Could you check a few things on this model? Use its own coordinates, in mm. Round coordinates to 2 decimals unless told otherwise and drop trailing zeros. Loops run counter-clockwise (first coordinate to the right, second up) from the corner with the lowest first, then second, coordinate; pieces in that order, holes last. Notation, with made-up numbers: (31.25, -25) - (69.25, -25) arc R28 ccw to (69.25, 13) - close; hole circle Ø7 at (-30.75, 13). An arc over 180 degrees is marked (long way). Answer as CSV lines item,"result". Start each with the question number.
1) Suppose I cut it at D-D, the plane z = 4.25. Write out the boundary of the cut face in (x, y), then the cut area to 3 significant figures.
2) Please list where these lines run through material, in increasing order: line 1 along Y through (x, z) = (0, 2); line 2 along Y through (x, z) = (-40, 5.75); line 3 along Y through (x, z) = (-33.02, 2.25).
3) We'd pull the mould along Y, two halves only. Please class faces 1 (the face through (0.425, -72.964, 3.131)), 2 (the face through (-37, 12.7, 3)), 3 (the face through (12.7, -39, 3)), 4 (the face through (0, -88.9, 3)): pulls with the +Y half, pulls with the -Y half, needs draft (parallel to the pull), parting line crosses it, or undercut.
4) Suppose I cut it at A-A, the plane x = -76.2. Write out the boundary of the cut face in (y, z), then the cut area to 3 significant figures.
5) Suppose I cut it at C-C, the plane y = 0. Write out the boundary of the cut face in (x, z), then the cut area to 3 significant figures.
6) I'm going to push flat-ended pins straight in: pin 1 Ø17.5 at (x, y) = (-33.02, -33.02) entering from -Z; pin 2 Ø2 at (y, z) = (-17.5, 5) entering from -X. Where does each tip first touch, or does it pass through?
7) Suppose I cut it at B-B, the plane y = -33.02. Write out the boundary of the cut face in (x, z), then the cut area to 3 significant figures.
```python
from build123d import *

# Parameters (mm, degrees)
SKETCH1_R               = 10.9855
BOSS_EXTRUDE1_DEPTH     = 6.35
F_1_4_CLEARANCE_HOLE1_D = 6.5278


with BuildPart() as part:
    # Sketch1 → Boss-Extrude1 (new body)
    with BuildSketch(Plane.XY):
        Polygon((-88.9, 12.7), (-88.9, -12.7), (-12.7, -88.9), (12.7, -88.9), (12.7, 12.7), align=None)
        with Locations((-33.02, -33.02)):
            Circle(SKETCH1_R, mode=Mode.SUBTRACT)
    extrude(amount=BOSS_EXTRUDE1_DEPTH)

    # 1/4 Clearance Hole1 (through all)
    with Locations(Plane.XY.offset(6.35)):
        with Locations((0, 0), (-76.2, 0), (0, -76.2)):
            Hole(F_1_4_CLEARANCE_HOLE1_D / 2)


solid = part.part
```
Filled sheet:
1,outline,"(-88.9, -12.7) - (-12.7, -88.9) - (12.7, -88.9) - (12.7, 12.7) - (-88.9, 12.7) - close; hole circle Ø6.53 at (-76.2, 0); hole circle Ø21.97 at (-33.02, -33.02); hole circle Ø6.53 at (0, -76.2); hole circle Ø6.53 at (0, 0)"
1,area,"6,940 mm²"
2,line 1,"-88.9 to -79.46, -72.94 to -3.26, 3.26 to 12.7"
2,line 2,"-61.6 to -41.5, -24.54 to 12.7"
2,line 3,"-68.58 to -44.01, -22.03 to 12.7"
3,face 1,"undercut"
3,face 2,"pulls with the +Y half"
3,face 3,"needs draft"
3,face 4,"pulls with the -Y half"
4,outline,"(-25.4, 0) - (-3.26, 0) - (-3.26, 6.35) - (-25.4, 6.35) - close; (3.26, 0) - (12.7, 0) - (12.7, 6.35) - (3.26, 6.35) - close"
4,area,"200 mm²"
5,outline,"(-88.9, 0) - (-79.46, 0) - (-79.46, 6.35) - (-88.9, 6.35) - close; (-72.94, 0) - (-3.26, 0) - (-3.26, 6.35) - (-72.94, 6.35) - close; (3.26, 0) - (12.7, 0) - (12.7, 6.35) - (3.26, 6.35) - close"
5,area,"562 mm²"
6,pin 1,"through"
6,pin 2,"x = -85.1"
7,outline,"(-68.58, 0) - (-44.01, 0) - (-44.01, 6.35) - (-68.58, 6.35) - close; (-22.03, 0) - (12.7, 0) - (12.7, 6.35) - (-22.03, 6.35) - close"
7,area,"377 mm²"
